from build123d import *

# Parameters (mm, degrees)
SKETCH4_W                                = 635
SKETCH4_H                                = 139.7
DIMENSIONS_CONTROL_OPTICS_LOCATION_DEPTH = 4
FILLET1_R                                = 1.27


with BuildPart() as part:
    # Sketch4 → DIMENSIONS CONTROL OPTICS LOCATION (new body)
    with BuildSketch(Plane.XY):
        with Locations((317.5, 69.85)):
            Rectangle(SKETCH4_W, SKETCH4_H)
        with BuildLine():
            Line((6.35, 93.996304065), (6.35, 45.703695935))
            ThreePointArc((6.35, 45.703695935), (56.604, 14.096), (106.858, 45.703695935))
            Line((106.858, 45.703695935), (106.985, 45.703695935))
            ThreePointArc((106.985, 45.703695935), (157.239, 14.096), (207.493, 45.703695935))
            Line((207.493, 45.703695935), (207.62, 45.703695935))
            ThreePointArc((207.62, 45.703695935), (257.874, 14.096), (308.128, 45.703695935))
            Line((308.128, 45.703695935), (308.255, 45.703695935))
            ThreePointArc((308.255, 45.703695935), (358.509, 14.096), (408.763, 45.703695935))
            Line((408.763, 45.703695935), (408.89, 45.703695935))
            ThreePointArc((408.89, 45.703695935), (459.144, 14.096), (509.398, 45.703695935))
            Line((509.398, 45.703695935), (509.525, 45.703695935))
            ThreePointArc((509.525, 45.703695935), (559.779, 14.096), (610.033, 45.703695935))
            Line((610.033, 45.703695935), (610.033, 93.996304065))
            ThreePointArc((610.033, 93.996304065), (559.779, 125.604), (509.525, 93.996304065))
            Line((509.525, 93.996304065), (509.398, 93.996304065))
            ThreePointArc((509.398, 93.996304065), (459.144, 125.604), (408.89, 93.996304065))
            Line((408.89, 93.996304065), (408.763, 93.996304065))
            ThreePointArc((408.763, 93.996304065), (358.509, 125.604), (308.255, 93.996304065))
            Line((308.255, 93.996304065), (308.128, 93.996304065))
            ThreePointArc((308.128, 93.996304065), (257.874, 125.604), (207.62, 93.996304065))
            Line((207.62, 93.996304065), (207.493, 93.996304065))
            ThreePointArc((207.493, 93.996304065), (157.239, 125.604), (106.985, 93.996304065))
            Line((106.985, 93.996304065), (106.858, 93.996304065))
            ThreePointArc((106.858, 93.996304065), (56.604, 125.604), (6.35, 93.996304065))
        make_face(mode=Mode.SUBTRACT)
    extrude(amount=DIMENSIONS_CONTROL_OPTICS_LOCATION_DEPTH)

    # Fillet1
    fillet1_edges = [part.edges().sort_by_distance(p)[0] for p in [
        (635, 0, 2),
        (0, 0, 2),
        (0, 139.7, 2),
        (635, 139.7, 2),
    ]]
    fillet(fillet1_edges, radius=FILLET1_R)


solid = part.part
Geometry check sheet. Reference: the model listing, model coordinates, mm. A direction names the side the tool comes from. Round coordinates to 2 decimals unless told otherwise and drop trailing zeros. Order: outer loops, then holes, each group sorted by start corner. A loop starts at its lowest first (then second) coordinate and runs counter-clockwise, first axis right, second up. Notation, with made-up numbers: M 13.5,24 L 35.5,24 A27 cw 35.5,52 Z; hole C -23.5,21 d3. An arc over 180 degrees is marked long. Answer in a Markdown table with one row per item. Add a question column.
Item 1: Sectioned sample at C-C, the plane y = 20. Enter the section's corners in (x, z).
Item 2: Material ranges on L1, parallel to X at y = 83.5, z = 1; L2, parallel to Y at x = 456, z = 0.6; L3, parallel to Y at x = 498, z = 0.6, recorded low to high. Write a range as [from, to].
Item 3: Sectioned sample at D-D, the plane x = 161. Enter the section's corners in (y, z), plus the area to 3 significant figures.
Item 4: Set-up check for faces 1 (the face through (316, 106.4, 4)), 2 (the face through (158.115, 125.597, 1.972)): record each of +Z, -Z, +X, -X, +Y, -Y from which the full face is reachable in a straight line by a thin tool's end or side.
Item 5: Draft check along X on faces 3 (the face through (316, 106.4, 0)), 4 (the face through (458.268, 14.103, 1.972)). Enter one of: released by +X, released by -X, zero draft, split by the parting line, or undercut.
Item 6: Sectioned sample at B-B, the plane x = 449.5. Enter the section's corners in (y, z), plus the area to 3 significant figures.
Filled in:
| question | item | result |
|---|---|---|
| 1 | outline | M 0,0 L 31.63,0 L 31.63,4 L 0,4 Z; M 81.57,0 L 132.27,0 L 132.27,4 L 81.57,4 Z; M 182.21,0 L 232.9,0 L 232.9,4 L 182.21,4 Z; M 282.84,0 L 333.54,0 L 333.54,4 L 282.84,4 Z; M 383.48,0 L 434.17,0 L 434.17,4 L 383.48,4 Z; M 484.11,0 L 534.81,0 L 534.81,4 L 484.11,4 Z; M 584.75,0 L 635,0 L 635,4 L 584.75,4 Z |
| 2 | L1 | x = [0, 6.35], [610.03, 635] |
| 2 | L2 | y = [0, 14.18], [125.52, 139.7] |
| 2 | L3 | y = [0, 29.87], [109.83, 139.7] |
| 3 | outline | M 0,0 L 14.22,0 L 14.22,4 L 0,4 Z; M 125.48,0 L 139.7,0 L 139.7,4 L 125.48,4 Z |
| 3 | area | 114 mm² |
| 4 | face 1 | +Z, +X, -X, +Y, -Y |
| 4 | face 2 | +Z, -Z |
| 5 | face 3 | zero draft |
| 5 | face 4 | undercut |
| 6 | outline | M 0,0 L 14.94,0 L 14.94,4 L 0,4 Z; M 124.76,0 L 139.7,0 L 139.7,4 L 124.76,4 Z |
| 6 | area | 119 mm² |
